```python
from build123d import *

# Parameters (mm, degrees)
BOSS_EXTRUDE1_DEPTH        = 12.7
CUT_EXTRUDE1_DEPTH         = 270.1976912701424
F_8_CLEARANCE_HOLE1_D      = 4.5
F_1_4_CLEARANCE_HOLE1_D    = 6.6
F_12_CLEARANCE_HOLE1_D     = 6
HOLE1_D                    = 6.4
HOLE1_DEPTH                = 24.77643101
HOLE1_CBORE_D              = 11.2
HOLE1_CBORE_DEPTH          = 11.77643101
F_10_CLEARANCE_HOLE1_D     = 5
F_10_CLEARANCE_HOLE1_DEPTH = 36.4125
CHAMFER1_SIZE              = 3.0000000000270917
SKETCH14_R                 = 2.9999999999999645
SKETCH14_R_2               = 1.6510000000000182
BOSS_EXTRUDE2_DEPTH        = 12.7
FILLET_1_R                 = 10
CUT_EXTRUDE_1_DEPTH        = 270.1976913300265
CUT_EXTRUDE_1_DEPTH_BACK   = 270.1976913300265
CUT_EXTRUDE_2_DEPTH        = 270.1976913300265


with BuildPart() as part:
    # Sketch1 → Boss-Extrude1 (new body)
    with BuildSketch(Plane(origin=(0, 0, 0), x_dir=(-1, 0, 0), z_dir=(0, 0, -1))):
        with BuildLine():
            Line((224.16945546503186, 127.72254562005153), (151.435240745465, 147.21161971627112))
            ThreePointArc((151.435240745465, 147.21161971627112), (105.25775385063858, 121.60745801933766), (129.24653278741587, 74.57053765621215))
            Line((129.24653278741587, 74.57053765621215), (211.46945546503187, 46.304993077870854))
            Line((211.46945546503187, 46.304993077870854), (224.16945546503186, 46.304993077870854))
            Line((224.16945546503186, 46.304993077870854), (224.16945546503186, 127.72254562005153))
        make_face()
    extrude(amount=-BOSS_EXTRUDE1_DEPTH)

    # Sketch2 → Cut-Extrude1 (cut, through all)
    with BuildSketch(Plane.XY.offset(12.7)):
        with BuildLine():
            Line((-103.63329146305492, 112.0939383172865), (-113.17901851462243, 112.0939383172865))
            ThreePointArc((-113.17901851462243, 112.0939383172865), (-113.13471703156931, 110.50643831728651), (-113.17901851462243, 108.9189383172865))
            Line((-113.17901851462243, 108.9189383172865), (-103.6332914630549, 108.91893831728652))
            ThreePointArc((-103.6332914630549, 108.91893831728652), (-103.60011703156931, 110.50643831728651), (-103.63329146305492, 112.0939383172865))
        make_face()
    extrude(amount=-CUT_EXTRUDE1_DEPTH, mode=Mode.SUBTRACT)

    # Sketch3 → Cut-Revolve1 (revolve, cut)
    with BuildSketch(Plane(origin=(0, 110.50643831728648, 0), x_dir=(1, 0, 0), z_dir=(0, 1, 0))):
        Polygon((-113.02511703156932, 3.5e-15), (-141.60011703156934, 0), (-141.60011703156934, -12.7), (-113.02511703156932, -12.7), align=None)
    revolve(axis=Axis((-141.60011703156934, 110.50643831728648, 0), (0, 0, 1)), mode=Mode.SUBTRACT)

    # #8 Clearance Hole1 (through all)
    with Locations(Plane.XY.offset(12.7)):
        with Locations((-117.978117032, 86.884438317), (-165.222117032, 86.884438317), (-165.222117032, 134.128438317), (-117.978117032, 134.128438317)):
            Hole(F_8_CLEARANCE_HOLE1_D / 2)

    # 1/4 Clearance Hole1 (through all)
    with Locations(Plane(origin=(0, 0, 0), x_dir=(-1, 0, 0), z_dir=(0, 0, -1))):
        with Locations((217.819455465, 53.304993078), (217.819455465, 76.304993078), (217.819455465, 99.304993078)):
            Hole(F_1_4_CLEARANCE_HOLE1_D / 2)

    # #12 Clearance Hole1 (through all)
    with Locations(Plane.XY.offset(12.7)):
        with Locations((-192.169455465, 89.72254562)):
            Hole(F_12_CLEARANCE_HOLE1_D / 2)

    # Hole1
    with Locations(Plane(origin=(0, 84.14250730723957, 0), x_dir=(-1, 0, 0), z_dir=(0, -1, 0))):
        with Locations((108.633291463, -6.35)):
            CounterBoreHole(HOLE1_D / 2, HOLE1_CBORE_D / 2, HOLE1_CBORE_DEPTH, depth=HOLE1_DEPTH)

    # #10 Clearance Hole1
    with Locations(Plane(origin=(0, 112.0939383172865, 0), x_dir=(-1, 0, 0), z_dir=(0, -1, 0))):
        with Locations((108.633291463, -6.35)):
            Hole(F_10_CLEARANCE_HOLE1_D / 2, depth=F_10_CLEARANCE_HOLE1_DEPTH)

    # Chamfer1
    chamfer1_edges = [part.edges().sort_by_distance(p)[0] for p in [
        (-221.11945546500002, 99.304993078, 0),
        (-221.11945546500002, 76.304993078, 0),
        (-221.11945546500002, 53.304993078, 0),
    ]]
    chamfer(chamfer1_edges, length=CHAMFER1_SIZE)

    # Sketch14 → Boss-Extrude2 (add)
    with BuildSketch(Plane(origin=(0, 0, 0), x_dir=(-1, 0, 0), z_dir=(0, 0, -1))):
        with Locations((192.16945546503186, 89.72254562005152)):
            Circle(SKETCH14_R)
        with Locations((192.16945546503186, 89.72254562005152)):
            Circle(SKETCH14_R_2, mode=Mode.SUBTRACT)
    extrude(amount=-BOSS_EXTRUDE2_DEPTH)

    # 圆角1
    fillet_1_edges = [part.edges().sort_by_distance(p)[0] for p in [
        (-224.16945546503186, 127.72254562005153, 6.35),
    ]]
    fillet(fillet_1_edges, radius=FILLET_1_R)

    # 草图1 → 切除-拉伸1 (cut, two sides: drawn at the far end of the back side and taken through both)
    with BuildSketch(Plane(origin=(0, 0, 0), x_dir=(-1, 0, 0), z_dir=(0, 0, -1)).offset(-CUT_EXTRUDE_1_DEPTH_BACK)):
        with BuildLine():
            Line((499.3977697015972, 53.97534108618588), (216.75764591605704, 129.7085340031526))
            Line((216.75764591605704, 129.7085340031526), (200.08107443086368, 134.17700786512998))
            ThreePointArc((200.08107443086368, 134.17700786512998), (217.45343902449696, 122.56916495351871), (224.16945546503186, 102.78441851073525))
            Line((224.16945546503186, 102.78441851073525), (224.16945546503186, 120.04927574026192))
            Line((224.16945546503186, 120.04927574026192), (224.16945546503186, 412.65986352358874))
            Line((224.16945546503186, 412.65986352358874), (-240.11771897993546, 56.399784399468274))
            Line((-240.11771897993546, 56.399784399468274), (35.11059525662989, -302.2847380379346))
            Line((35.11059525662989, -302.2847380379346), (499.3977697015972, 53.97534108618588))
        make_face()
    extrude(amount=CUT_EXTRUDE_1_DEPTH + CUT_EXTRUDE_1_DEPTH_BACK, mode=Mode.SUBTRACT)

    # 草图2 → 切除-拉伸2 (cut, through all)
    with BuildSketch(Plane(origin=(0, 0, 0), x_dir=(-1, 0, 0), z_dir=(0, 0, -1))):
        Polygon((171.07059959298968, 70.76717861409958), (204.1694554650319, 59.388877336589836), (193.30917816776565, 81.6274559113658), align=None)
        Polygon((181.27084732320867, 112.69613365514031), (173.24474011566244, 131.01502016859888), (204.1694554650319, 122.72876766457311), align=None)
    extrude(amount=-CUT_EXTRUDE_2_DEPTH, mode=Mode.SUBTRACT)


solid = part.part
```
For this review, take the finished solid that the model builds, in its own axes (mm). A direction names the side the tool comes from. Give positions to 0.01 mm unless a question says otherwise; leave off trailing zeros. Write each loop counter-clockwise with the first axis right and the second up, starting at its lowest first coordinate (ties: lowest second). Pieces come first, ordered by that corner, then holes.
Item 1: Take a section at A-A (y = 107.5). Give the boundary of the cut face in (x, z).
Item 2: Take a section at C-C (x = -138). Give the boundary of the cut face in (y, z), and give its area (3 significant figures).
Item 3: Take a section at B-B (z = 6.35). Give the number of separate pieces and of enclosed holes in the cut face, and give its area (3 significant figures).
Item 4: Wall thickness on probe 1 along Y at (x, z) = (-116, 7.25); probe 2 along Y at (x, z) = (-166, 4); probe 3 along X at (y, z) = (116, 10.25): over which ranges is each line inside the solid? List them lowest first.
Item 5: The part is to be moulded in two halves that separate along X. For faces 1 (the face through (-169.782, 60.636, 6.261)), 2 (the face through (-119.49, 141.41, 6.26)), 3 (the face through (-182.346, 76.273, 6.261)), say which applies: +X half, -X half, draft (parallel to the pull), parting line (faces both ways), or undercut.
Item 6: Machinability: for faces 4 (the face through (-105, 108.919, 6)), 5 (the face through (-216.05, 102.09, 7.92)), which of the approach directions +Z, -Z, +X, -X, +Y, -Y give a long, thin tool a straight path to every point of the face, cutting with its end or side? Answer none if there is none.
Item 7: Insertion check: P1, Ø5, axis at x = -168, z = 10, coming from the +Y side; P2, Ø4, axis at x = -115.5, z = 7, coming from the +Y side; P3, Ø6, axis at x = -217.82, y = 53.3, coming from the +Z side; P4, Ø6.5, axis at x = -108.63, z = 6.35, coming from the +Y side. Each pin has a flat end and moves straight along its axis. Give the tip position at first contact, or say it passes through.
Established:
1. outline: (-223.83, 0) - (-170.02, 0) - (-170.02, 12.7) - (-223.83, 12.7) - close; (-113.18, 0) - (-103.72, 0) - (-103.72, 12.7) - (-113.18, 12.7) - close; hole circle Ø6.4 at (-108.63, 6.35)
2. outline: (71.56, 0) - (82.16, 0) - (82.16, 12.7) - (71.56, 12.7) - close; (138.85, 0) - (148.34, 0) - (148.34, 12.7) - (138.85, 12.7) - close
2. area: 255 mm2
3. separate pieces: 3
3. enclosed holes: 10
3. area: 5,410 mm2
4. probe 1: y = 82.42 to 85.81, 87.96 to 97.81, 123.2 to 133.06, 135.2 to 138.59
4. probe 2: y = 61.94 to 84.77, 89 to 95.63, 125.38 to 132.02, 136.24 to 143.31
4. probe 3: x = -221.36 to -188.81, -179.82 to -169.64, -113.56 to -104
5. face 1: +X half
5. face 2: parting line
5. face 3: undercut
6. face 4: +Z, -Z, +X
6. face 5: +Z, -Z
7. P1: stops at y = 143.44
7. P2: stops at y = 139.89
7. P3: passes through
7. P4: stops at y = 134.19
